Print and shaded views of the part. All mm, measured from the part's lowest x, y and z. A direction names the side the tool comes from. Round coordinates to 2 decimals unless told otherwise and drop trailing zeros. Order: outer loops, then holes, each group sorted by start corner. A loop starts at its lowest first (then second) coordinate and runs counter-clockwise, first axis right, second up.
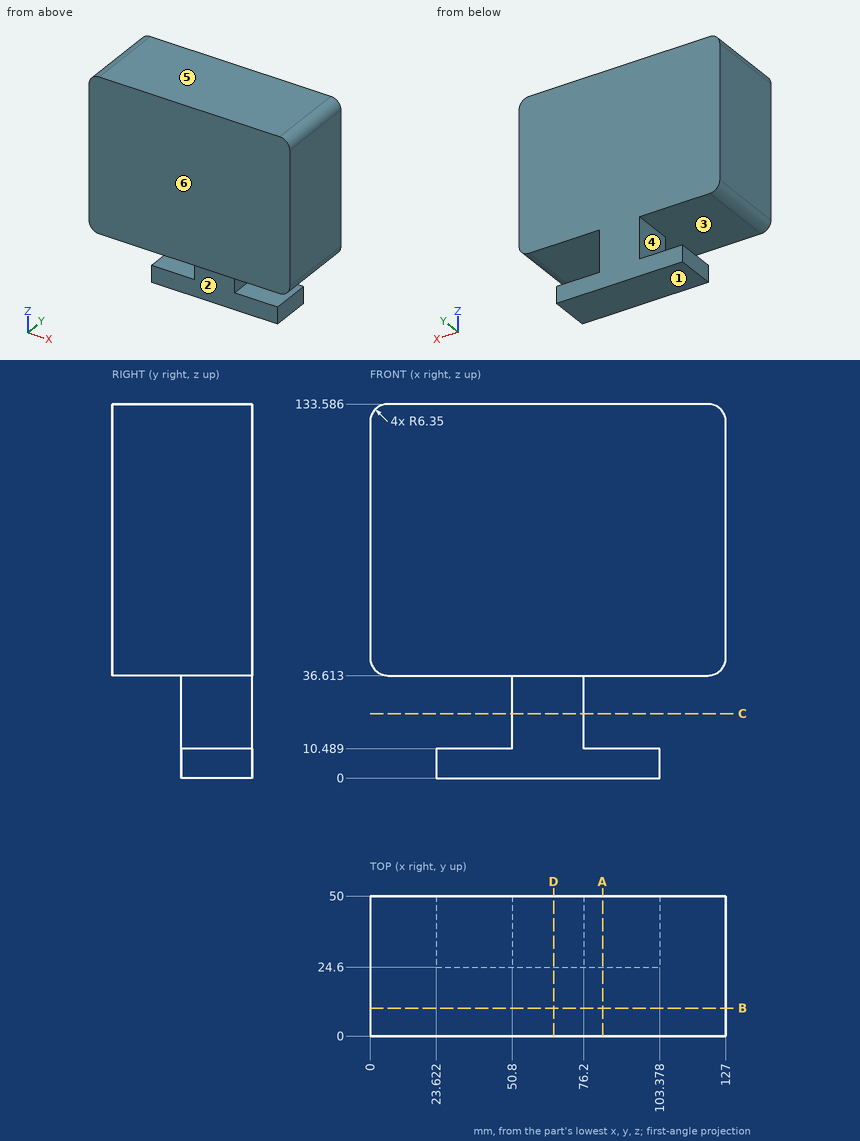
1. Cut at D-D, the plane x = 65.5. Write the cut outline in (y, z).
2. Tool access for the marked faces 1 and 2: list every direction of +Z, -Z, +X, -X, +Y, -Y with a clear straight run to the whole face (end or side of a thin tool).
3. Cut at B-B, the plane y = 10. Write the cut outline in (x, z), and give its area (3 significant figures).
4. Drill centre lines: line 1 (Z direction, x = 39, y = 34); line 2 (Z direction, x = 9, y = 41); line 3 (X direction, y = 22, z = 127.5) (1 decimal). Where is each one in solid material? Low to high.
5. Pin check, flat tips, straight feed: P1, Ø11.5, axis at y = 32.5, z = 5, coming from the +X side; P2, Ø1, axis at y = 40.5, z = 41.5, coming from the +X side; P3, Ø11, axis at x = 57, z = 24.5, coming from the -Y side. Stop position of each tip, or through.
6. Mould opens along Z. For the marked faces 3, 4, 5 and 6 say: released by +Z, released by -Z, zero draft, split by the parting line, or undercut.
7. Cut at A-A, the plane x = 83. Write the cut outline in (y, z).
8. Cut at C-C, the plane z = 23. Write the cut outline in (x, y), and give its area (3 significant figures).
Outcome:
1. outline: (0, 36.61) - (24.6, 36.61) - (24.6, 0) - (50, 0) - (50, 133.59) - (0, 133.59) - close
2. face 1: -Z, +X, -X, +Y, -Y
2. face 2: -Z, +X, -X, -Y
3. outline: (0, 42.96) arc R6.35 ccw to (6.35, 36.61) - (120.65, 36.61) arc R6.35 ccw to (127, 42.96) - (127, 127.24) arc R6.35 ccw to (120.65, 133.59) - (6.35, 133.59) arc R6.35 ccw to (0, 127.24) - close
3. area: 12,300 mm2
4. line 1: z = 0 to 10.49, 36.61 to 133.59
4. line 2: z = 36.61 to 133.59
4. line 3: x = 0 to 127
5. P1: stops at x = 103.38
5. P2: stops at x = 126.93
5. P3: stops at y = 24.6
6. face 3: undercut
6. face 4: undercut
6. face 5: released by +Z
6. face 6: zero draft
7. outline: (0, 36.61) - (50, 36.61) - (50, 133.59) - (0, 133.59) - close; (24.6, 0) - (50, 0) - (50, 10.49) - (24.6, 10.49) - close
8. outline: (50.8, 24.6) - (76.2, 24.6) - (76.2, 50) - (50.8, 50) - close
8. area: 645 mm2
